CAD build for the part. Positions are in the model's coordinates, mm. Face numbers are marked on the shaded views. Coordinates: 2 decimals unless noted, no trailing zeros. Write each loop counter-clockwise with the first axis right and the second up, starting at its lowest first coordinate (ties: lowest second). Pieces come first, ordered by that corner, then holes. Notation, with made-up numbers: (35.5, 23) - (90.5, 23) arc R29 ccw to (90.5, 47) - close; hole circle Ø6 at (-13, 40.5). An arc over 180 degrees is marked (long way). Answer in a Markdown table with one row per item. Add a question column.
Q1. Pin check, flat tips, straight feed: pin 1 (1 mm diameter, centred on y = 0, z = 2, fed in from -X); pin 2 (1 mm diameter, centred on x = -0.5, z = -1.5, fed in from -Y); pin 3 (0.9 mm diameter, centred on x = 0, z = 4.5, fed in from -Y). Stop position of each tip, or through.
Q2. Two-plate mould, pull along Y, no slides. Class the marked faces 1, 2 and 3: +Y half, -Y half, draft (parallel to the pull), parting line (faces both ways), or undercut.
Q3. Band-saw the part on A-A (z = -2). List the corners of the cut face in (x, y).
Q4. Drill centre lines: line 1 along Z through (x, y) = (0.5, -0.55); line 2 along Y through (x, z) = (0, 2.25); line 3 along Y through (x, z) = (1.1, 4.75). Where is each one in solid material? Low to high. Write a range as from..to.
Autodesk Inventor part; units mm, degrees
ref_plane "YZ Plane" through (0, 0, 0) normal (1, 0, 0) x (0, 1, 0)
ref_plane "XZ Plane" through (0, 0, 0) normal (0, 1, 0) x (-1, 0, 0)
ref_plane "XY Plane" through (0, 0, 0) normal (0, 0, 1) x (1, 0, 0)
sketch "Sketch1" plane through (0, 0, 0) normal (0, 1, 0) x (-1, 0, 0)
  line L0 (0, 4.2476) -> (0, -4.2476)
  line L1 (0, -4.2476) -> (-1.25, -4.2476)
  line L2 (-1.25, -4.2476) -> (-1.5, -3.9976)
  line L3 (-1.5, -3.9976) -> (-1.5, 3.6524)
  line L4 (-1.6, 3.7524) -> (-2.85, 3.7524)
  line L5 (-2.85, 3.7524) -> (-2.85, 4.0024)
  line L6 (0, 4.2476) -> (-1.1547, 5.4024)
  line L7 (-1.1547, 5.4024) -> (-1.5, 5.4024)
  arc A0 (-1.5, 5.4024) -> (-2.85, 4.0024) centre (0, 2.605) ccw
  line L8 (-1.1547, 5.4024) -> (-0.5774, 6.4024) construction
  line L9 (-0.5774, 6.4024) -> (0.5774, 6.4024) construction
  line L10 (0.5774, 6.4024) -> (1.1547, 5.4024) construction
  line L11 (1.1547, 5.4024) -> (0.5774, 4.4024) construction
  line L12 (0.5774, 4.4024) -> (-0.5774, 4.4024) construction
  line L13 (-0.5774, 4.4024) -> (-1.1547, 5.4024) construction
  arc A1 (-1.5, 3.6524) -> (-1.6, 3.7524) centre (-1.6, 3.6524) ccw
  point P0 (0, 0)
  point P1 (-1.5, 3.7524)
  point P2 (0, 0)
  point P3 (0, 5.4024)
  dimension "d0" = 3
  dimension "d1" = 8
  dimension "d2" = 0.25
  dimension "d3" = 135
  dimension "d4" = 5.7
  dimension "d5" = 3
  dimension "d6" = 1.65
  dimension "d7" = 2
  dimension "d8" = 0.25
  dimension "d15" = 3.2
revolve "Revolution1" add sketch "Sketch1" angle 360 about axis through (0, 0, 4.2476) along (0, 0, -1)
sketch "Sketch2" plane through (0, 0, 5.4024) normal (0, 0, 1) x (1, 0, 0)
  circle A0 centre (0, 0) radius 1.1547
  circle A1 centre (0, 0) radius 1.5
  line L0 (-1.1547, 0) -> (-0.5774, 1)
  line L1 (-0.5774, 1) -> (0.5774, 1)
  line L2 (0.5774, 1) -> (1.1547, 0)
  line L3 (1.1547, 0) -> (0.5774, -1)
  line L4 (0.5774, -1) -> (-0.5774, -1)
  line L5 (-0.5774, -1) -> (-1.1547, 0)
  point P0 (0, 0)
extrude "Extrusion1" cut sketch "Sketch2" against normal blind 1.2 contours L3 L4 L5 L0 L1 L2
thread "Thread1"
properties part number "48-0380" material "Stainless Steel"
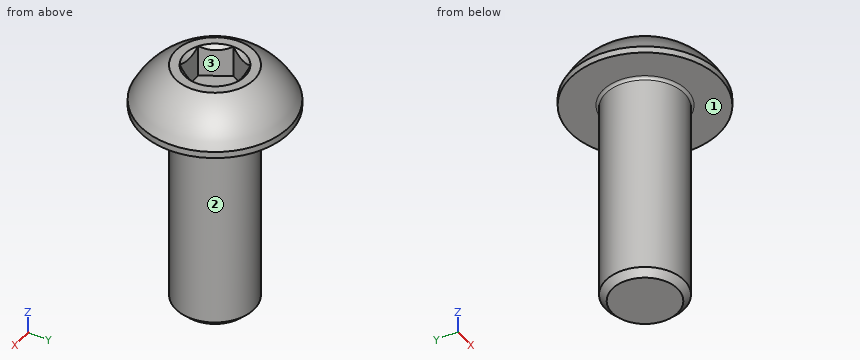
Checked values:
| question | item | result |
|---|---|---|
| 1 | pin 1 | stops at x = -1.5 |
| 1 | pin 2 | stops at y = -1.5 |
| 1 | pin 3 | stops at y = -2.83 |
| 2 | face 1 | draft |
| 2 | face 2 | parting line |
| 2 | face 3 | undercut |
| 3 | outline | circle Ø3 at (0, 0) |
| 4 | line 1 | z = -4.25..4.2 |
| 4 | line 2 | y = -1.5..1.5 |
| 4 | line 3 | y = -2.07..-0.09, 0.09..2.07 |
